Verification items for this drawing (mm, ordinates from the low corner). A direction names the side the tool comes from. Coordinates: 2 decimals unless noted, no trailing zeros. Loops run counter-clockwise (first coordinate to the right, second up) from the corner with the lowest first, then second, coordinate; pieces in that order, holes last. Notation, with made-up numbers: (-23.75, 19) - (15.25, 19) arc R6 cw to (15.25, 25) - close; hole circle Ø4 at (-30.5, -5). An arc over 180 degrees is marked (long way). Write each question's results on one line, items separated by ' | '. Start each with the question number.
(1) Sectioned sample at B-B (z = 95). Enter the section's corners in (x, y) (1 decimal).
(2) Go/stop test with flat-tipped pins: pin 1 Ø5 at (x, y) = (70, 46.5) entering from +Z (1 decimal); pin 2 Ø8 at (x, y) = (104.5, 27) entering from -Z; pin 3 Ø10 at (x, y) = (62.5, 131.5) entering from +Z. Record where each tip stops, or that it passes through.
(3) Mould release check, pull along X, two halves, no side actions. Record for the marked faces 1, 2 and 3: pulls with the +X half, pulls with the -X half, needs draft (parallel to the pull), parting line crosses it, or undercut.
(4) Sectioned sample at C-C (x = 38.5). Enter the section's corners in (y, z), plus the area to 3 significant figures.
(5) Material ranges on probe 1 along X at (y, z) = (121, 94.5); probe 2 along Z at (x, y) = (112.5, 36) (1 decimal); probe 3 along Y at (x, z) = (30, 59), recorded low to high.
(6) Access from +Z, -Z, +X, -X, +Y, -Y to the whole of each face (thin tool, end or side, straight path). Record for the marked faces 4 and 5.
(7) Sectioned sample at A-A (y = 114.5). Enter the section's corners in (x, z).
(8) Sectioned sample at D-D (y = 73.5). Enter the section's corners in (x, z), plus the area to 3 significant figures.
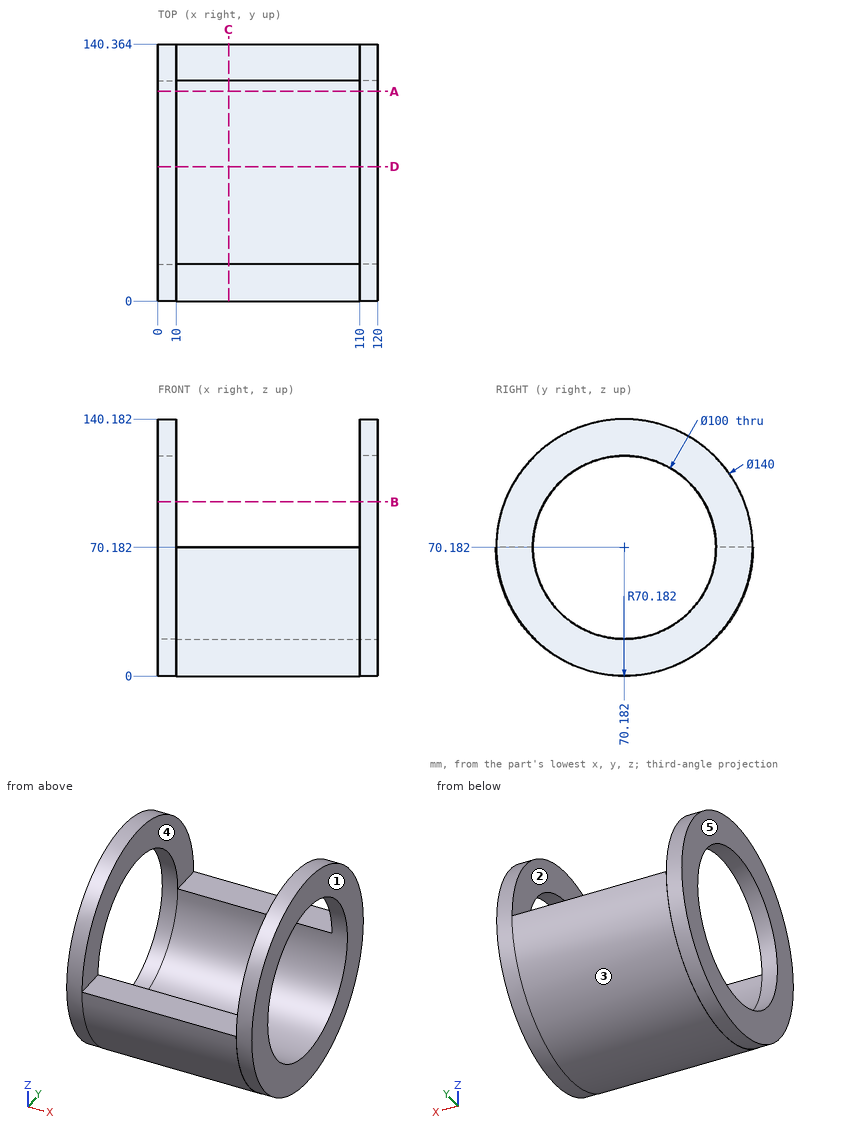
Outcome:
1) outline: (0, 4.7) - (10, 4.7) - (10, 26.8) - (0, 26.8) - close; (0, 113.6) - (10, 113.6) - (10, 135.6) - (0, 135.6) - close; (110, 4.7) - (120, 4.7) - (120, 26.8) - (110, 26.8) - close; (110, 113.6) - (120, 113.6) - (120, 135.6) - (110, 135.6) - close
2) pin 1: stops at z = 27.6 | pin 2: stops at z = 11.96 | pin 3: stops at z = 70.18
3) face 1: pulls with the +X half | face 2: undercut | face 3: needs draft
4) outline: (0, 70.18) arc R70.18 ccw to (140.36, 70.18) - (120.18, 70.18) arc R50 cw to (20.18, 70.18) - close | area: 3,810 mm2
5) probe 1: x = 0 to 10, 110 to 120 | probe 2: z = 9.1 to 33.7, 106.7 to 131.3 | probe 3: y = 0.9 to 21.45, 118.92 to 139.47
6) face 4: +Z, +Y, -Y | face 5: +Z, -Z, -X, +Y, -Y
7) outline: (0, 16) - (10, 16) - (10, 15.76) - (110, 15.76) - (110, 16) - (120, 16) - (120, 47.03) - (0, 47.03) - close; (0, 93.33) - (10, 93.33) - (10, 124.37) - (0, 124.37) - close; (110, 93.33) - (120, 93.33) - (120, 124.37) - (110, 124.37) - close
8) outline: (0, 0.26) - (10, 0.26) - (10, 0.08) - (110, 0.08) - (110, 0.26) - (120, 0.26) - (120, 20.29) - (0, 20.29) - close; (0, 120.07) - (10, 120.07) - (10, 140.1) - (0, 140.1) - close; (110, 120.07) - (120, 120.07) - (120, 140.1) - (110, 140.1) - close | area: 2,820 mm2
